Read the model definition and answer for the solid it produces. Units are mm, in the model's axes. Face numbers are marked on the shaded views. A direction names the side the tool comes from. Round coordinates to 2 decimals unless told otherwise and drop trailing zeros. Order: outer loops, then holes, each group sorted by start corner. A loop starts at its lowest first (then second) coordinate and runs counter-clockwise, first axis right, second up. Notation, with made-up numbers: (-37, -1) - (7, -1) arc R20 cw to (7, 12) - close; hole circle Ø6 at (-21.75, 51.5). An arc over 180 degrees is marked (long way). Put each result on its own line as item: value. Start each with the question number.
Q1. Each of these flat-tipped pins is pushed along its axis until it touches: pin 1 Ø6 at (x, y) = (-11, -3) entering from +Z; pin 2 Ø1.5 at (x, y) = (1, -18) entering from -Z; pin 3 Ø1.5 at (x, y) = (-20, -4) entering from +Z; pin 4 Ø1 at (x, z) = (1, 13) entering from -Y. Where does it stop, or does it pass through?
Q2. Which of the six approach directions +Z, -Z, +X, -X, +Y, -Y give full straight-line access (tool end or side, diameter ignored) to the marked faces 1 and 2?
Q3. Section B-B on y = 0 is taken. State how many separate pieces and enclosed holes the cut face has, then the cut area to 3 significant figures.
Q4. Section C-C on x = 1.5 is taken. Give the vertices of the cut face in (y, z).
Q5. Section A-A on z = 9.75 is taken. Give the vertices of the cut face in (x, y).
Q6. Find the intervals of material crossed by line 1 along X through (y, z) = (0, 4); line 2 along Y through (x, z) = (-18.3, 3.55); line 3 along X through (y, z) = (-23, 5.5), in increasing order. Write a range as from..to.
Q7. For a pull along Y with two mould halves and no side action, classify the marked faces 3, 4 and 5 as pulls with the +Y half, pulls with the -Y half, needs draft (parallel to the pull), parting line crosses it, or undercut.
Q8. Section D-D on y = 20.5 is taken. Give the vertices of the cut face in (x, z).
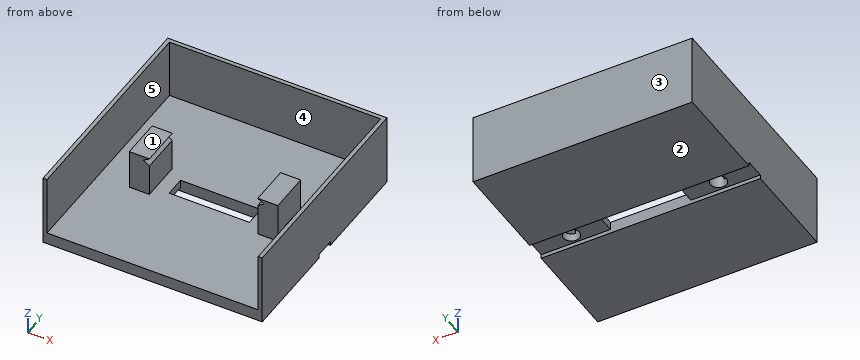
from build123d import *

# Parameters (mm, degrees)
SKICA1_W                 = 54.6
SKICA1_H                 = 54.6
P_IDAT_VYSUNUT_M2_DEPTH  = 3
SKICA4_W                 = 20
SKICA4_H                 = 5
ODEBRAT_VYSUNUT_M1_DEPTH = 2
SKICA5_W                 = 54.6
SKICA5_H                 = 5
ODEBRAT_VYSUNUT_M3_DEPTH = 1
SKICA10_W                = 5
SKICA10_H                = 10
P_IDAT_VYSUNUT_M6_DEPTH  = 10
ODEBRAT_VYSUNUT_M6_DEPTH = 10
P_IDAT_VYSUNUT_M9_DEPTH  = 15
SKICA17_R                = 2
ODEBRAT_VYSUNUT_M8_DEPTH = 4


with BuildPart() as part:
    # Skica1 → Přidat vysunutím2 (new body)
    with BuildSketch(Plane.XY):
        Rectangle(SKICA1_W, SKICA1_H)
    extrude(amount=P_IDAT_VYSUNUT_M2_DEPTH)

    # Skica4 → Odebrat vysunutím1 (cut)
    with BuildSketch(Plane.XY.offset(3)):
        Rectangle(SKICA4_W, SKICA4_H)
    extrude(amount=-ODEBRAT_VYSUNUT_M1_DEPTH, mode=Mode.SUBTRACT)

    # Skica5 → Odebrat vysunutím3 (cut)
    with BuildSketch(Plane(origin=(0, 0, 0), x_dir=(-1, 0, 0), z_dir=(0, 0, -1))):
        Rectangle(SKICA5_W, SKICA5_H)
    extrude(amount=-ODEBRAT_VYSUNUT_M3_DEPTH, mode=Mode.SUBTRACT)

    # Skica10 → Přidat vysunutím6 (add)
    with BuildSketch(Plane.XY.offset(3)):
        with Locations((-16, 0)):
            Rectangle(SKICA10_W, SKICA10_H)
        with Locations((16, 0)):
            Rectangle(SKICA10_W, SKICA10_H)
    extrude(amount=P_IDAT_VYSUNUT_M6_DEPTH)

    # Skica12 → Odebrat vysunutím6 (cut)
    with BuildSketch(Plane(origin=(0, 5, 0), x_dir=(1, 0, 0), z_dir=(0, 1, 0))):
        Polygon((-13.5, -13), (-13.5, -11), (-15, -12), align=None)
        Polygon((13.5, -13), (13.5, -11), (15, -12), align=None)
    extrude(amount=-ODEBRAT_VYSUNUT_M6_DEPTH, mode=Mode.SUBTRACT)

    # Skica14 → Přidat vysunutím9 (add)
    with BuildSketch(Plane.XY.offset(3)):
        Polygon((27.3, 27.3), (-27.3, 27.3), (-27.3, -27.3), (-26.3, -27.3), (-26.3, 26.3), (26.3, 26.3), (26.3, -27.3), (27.3, -27.3), align=None)
    extrude(amount=P_IDAT_VYSUNUT_M9_DEPTH)

    # Skica17 → Odebrat vysunutím8 (cut)
    with BuildSketch(Plane(origin=(0, 0, 1), x_dir=(-1, 0, 0), z_dir=(0, 0, -1))):
        with Locations((-18.3, 0)):
            Circle(SKICA17_R)
        with Locations((18.3, 0)):
            Circle(SKICA17_R)
    extrude(amount=-ODEBRAT_VYSUNUT_M8_DEPTH, mode=Mode.SUBTRACT)


solid = part.part
Findings:
1. pin 1: z = 13
1. pin 2: z = 0
1. pin 3: z = 3
1. pin 4: y = 26.3
2. face 1: +Z, -Y
2. face 2: -Z, +X, -X, +Y, -Y
3. separate pieces: 4
3. enclosed holes: 0
3. area: 171 mm2
4. outline: (-27.3, 0) - (-2.5, 0) - (-2.5, 3) - (-27.3, 3) - close; (2.5, 0) - (27.3, 0) - (27.3, 18) - (26.3, 18) - (26.3, 3) - (2.5, 3) - close
5. outline: (-27.3, -27.3) - (-26.3, -27.3) - (-26.3, 26.3) - (26.3, 26.3) - (26.3, -27.3) - (27.3, -27.3) - (27.3, 27.3) - (-27.3, 27.3) - close; (-18.5, -5) - (-13.5, -5) - (-13.5, 5) - (-18.5, 5) - close; (13.5, -5) - (18.5, -5) - (18.5, 5) - (13.5, 5) - close
6. line 1: -27.3..-26.3, -16.3..-13.5, 13.5..16.3, 26.3..27.3
6. line 2: -5..-2, 2..5, 26.3..27.3
6. line 3: -27.3..-26.3, 26.3..27.3
7. face 3: pulls with the +Y half
7. face 4: undercut
7. face 5: needs draft
8. outline: (-27.3, 0) - (27.3, 0) - (27.3, 18) - (26.3, 18) - (26.3, 3) - (-26.3, 3) - (-26.3, 18) - (-27.3, 18) - close
